from build123d import *

# Parameters (mm, degrees)
BOSS_EXTRUDE1_DEPTH         = 3.175
M3_CLEARANCE_HOLE1_D        = 3.6
F_1_4_CLEARANCE_HOLE1_D     = 7.14248
CUT_EXTRUDE1_DEPTH          = 640.11012417
F_8_CLEARANCE_HOLE1_D       = 4.9149
SKETCH15_R                  = 1.55
CUT_EXTRUDE2_DEPTH          = 640.11012417
SKETCH16_R                  = 3.3782
CUT_EXTRUDE3_DEPTH          = 640.11012417
FILLET1_R                   = 1
CUT_EXTRUDE4_DEPTH          = 640.088878697
FILLET2_R                   = 1.5
F_13_0_185_DIAMETER_HOLE1_D = 4.699
F_1_4_CLEARANCE_HOLE2_D     = 6.7564


with BuildPart() as part:
    # Sketch1 → Boss-Extrude1 (new, symmetric)
    with BuildSketch(Plane(origin=(0, 0, 0), x_dir=(1, 0, 0), z_dir=(0, 1, 0))):
        Polygon((0, -94.3735), (0, 94.3735), (-621.526239041, 148.75), (-621.526239041, -148.75), align=None)
    extrude(amount=BOSS_EXTRUDE1_DEPTH, both=True)

    # M3 Clearance Hole1 (through all)
    with Locations(Plane(origin=(0, 3.175, 0), x_dir=(1, 0, 0), z_dir=(0, 1, 0))):
        with Locations((-379.222, 34.29), (-384.81, 34.29), (-384.81, -34.29)):
            Hole(M3_CLEARANCE_HOLE1_D / 2)

    # 1/4 Clearance Hole1 (through all)
    with Locations(Plane(origin=(0, 3.175, 0), x_dir=(1, 0, 0), z_dir=(0, 1, 0))):
        with Locations((-29.147346667, 72.452653333), (-29.147346667, -72.452653333), (-148.652653333, -72.452653333), (-148.652653333, 72.452653333)):
            Hole(F_1_4_CLEARANCE_HOLE1_D / 2)

    # Sketch12 → Cut-Extrude1 (cut, through all)
    with BuildSketch(Plane(origin=(0, 3.175, 0), x_dir=(1, 0, 0), z_dir=(0, 1, 0))):
        with BuildLine():
            Line((-380.84125, -33.6169), (-380.84125, -34.0868))
            ThreePointArc((-380.84125, -34.0868), (-380.85395, -34.29), (-380.84125, -34.4932))
            Line((-380.84125, -34.4932), (-380.84125, -34.9631))
            ThreePointArc((-380.84125, -34.9631), (-379.222, -36.58235), (-377.60275, -34.9631))
            Line((-377.60275, -34.9631), (-377.60275, -34.4932))
            ThreePointArc((-377.60275, -34.4932), (-377.59005, -34.29), (-377.60275, -34.0868))
            Line((-377.60275, -34.0868), (-377.60275, -33.6169))
            ThreePointArc((-377.60275, -33.6169), (-379.222, -31.99765), (-380.84125, -33.6169))
        make_face()
    extrude(amount=-CUT_EXTRUDE1_DEPTH, mode=Mode.SUBTRACT)

    # #8 Clearance Hole1 (through all)
    with Locations(Plane(origin=(0, 3.175, 0), x_dir=(1, 0, 0), z_dir=(0, 1, 0))):
        with Locations((-508.833140591, -78.064272283), (-508.833140591, -103.464272283), (-543.213396712, -112.444528404), (-534.233140591, -78.064272283), (-481.407885674, -78.064272283), (-481.407885674, -103.464272283), (-456.007885674, -78.064272283), (-456.007885674, -103.464272283), (-456.007885674, 78.064272283), (-456.007885674, 103.464272283), (-481.407885674, 78.064272283), (-481.407885674, 103.464272283), (-543.213396712, 112.444528404), (-534.233140591, 78.064272283), (-508.833140591, 103.464272283), (-508.833140591, 78.064272283)):
            Hole(F_8_CLEARANCE_HOLE1_D / 2)

    # Sketch15 → Cut-Extrude2 (cut, through all)
    with BuildSketch(Plane(origin=(0, 3.175, 0), x_dir=(1, 0, 0), z_dir=(0, 1, 0))):
        with Locations(Location((-295.918163181, -81.916960017, 0), (0, 0, 270))):
            Circle(SKETCH15_R)
        with Locations(Location((-364.1575, -87.887128395, 0), (0, 0, 270))):
            Circle(SKETCH15_R)
    extrude(amount=-CUT_EXTRUDE2_DEPTH, mode=Mode.SUBTRACT)

    # Sketch16 → Cut-Extrude3 (cut, through all)
    with BuildSketch(Plane(origin=(0, 3.175, 0), x_dir=(1, 0, 0), z_dir=(0, 1, 0))):
        with Locations(Location((-609.6000104, -121.650317511, 0), (0, 0, 270))):
            Circle(SKETCH16_R)
        with Locations(Location((-609.6000104, -86.943080709, 0), (0, 0, 270))):
            Circle(SKETCH16_R)
        with Locations(Location((-609.6000104, 86.943080709, 0), (0, 0, 270))):
            Circle(SKETCH16_R)
        with Locations(Location((-609.6000104, 121.650317511, 0), (0, 0, 270))):
            Circle(SKETCH16_R)
    extrude(amount=-CUT_EXTRUDE3_DEPTH, mode=Mode.SUBTRACT)

    # Fillet1
    fillet1_edges = [part.edges().sort_by_distance(p)[0] for p in [
        (-621.526239041, 0, 148.75),
        (-621.526239041, 0, -148.75),
    ]]
    fillet(fillet1_edges, radius=FILLET1_R)

    # Sketch17 → Cut-Extrude4 (cut, through all)
    with BuildSketch(Plane(origin=(0, 3.175, 0), x_dir=(1, 0, 0), z_dir=(0, 1, 0))):
        Polygon((-3, 94.635965991), (-3, 59.635965991), (0, 59.635965991), (0, 94.3735), align=None)
    cut_extrude4 = extrude(amount=-CUT_EXTRUDE4_DEPTH, mode=Mode.SUBTRACT)

    # Mirror1: Cut-Extrude4 across plane
    add(cut_extrude4.mirror(Plane.XY), mode=Mode.SUBTRACT)

    # Fillet2
    fillet2_edges = [part.edges().sort_by_distance(p)[0] for p in [
        (0, 0, -59.635965991),
        (-3, 0, -59.635965991),
        (-3, 0, -94.635965991),
        (0, 0, 59.635965991),
        (-3, 0, 59.635965991),
        (-3, 0, 94.635965991),
    ]]
    fillet(fillet2_edges, radius=FILLET2_R - 0.0001)  # a hair under: the kernel refuses the full size

    # #13 (0.185) Diameter Hole1 (through all)
    with Locations(Plane(origin=(0, 3.175, 0), x_dir=(1, 0, 0), z_dir=(0, 1, 0))):
        with Locations((-354.44558465, 73.187743603), (-304.635849746, 68.829956465)):
            Hole(F_13_0_185_DIAMETER_HOLE1_D / 2)

    # 1/4 Clearance Hole2 (through all)
    with Locations(Plane(origin=(0, 3.175, 0), x_dir=(1, 0, 0), z_dir=(0, 1, 0))):
        with Locations((-14.732, 88.469940408), (-14.0462, -87.453940528), (-303.7332, 0)):
            Hole(F_1_4_CLEARANCE_HOLE2_D / 2)


solid = part.part
Build history of the part. All positions in model axes, mm. Round coordinates to 2 decimals unless told otherwise and drop trailing zeros. Loops run counter-clockwise (first coordinate to the right, second up) from the corner with the lowest first, then second, coordinate; pieces in that order, holes last. Notation, with made-up numbers: (31.25, 14.25) -> (63.25, 14.25) arc R23 cw to (63.25, 39.25) -> close; hole circle Ø3 at (-7, 26.5). An arc over 180 degrees is marked (long way). Use CSV: the item, a comma, the result in double quotes. Start each with the question number.
Q1. Saw through at A-A on y = -0.5. Count the separate pieces of the cut face and the enclosed holes in it, and give its area (3 significant figures).
Q2. Drill centre lines: L1, parallel to X at y = 0, z = 35.5; L2, parallel to Z at x = -131, y = 1; L3, parallel to Z at x = -286.5, y = 2.5. Where is each one in solid material? Low to high.
Q3. Flat gauge pins, fed straight in: pin 1 Ø2 at (x, y) = (-70.5, -2) entering from +Z; pin 2 Ø8 at (x, z) = (-481.41, 78.06) entering from -Y (3 decimals); pin 3 Ø3 at (x, y) = (-515.5, -0.5) entering from -Z; pin 4 Ø3 at (y, z) = (0, -81.5) entering from +X. Where does each tip first touch, or does it go through?
Q4. Mould opens along X. For faces 1 (the face through (-316.717, 0.044, 122.083)), 2 (the face through (-315, 3.175, -2)) say: +X half, -X half, draft (parallel to the pull), parting line (faces both ways), or undercut.
Q5. Saw through at B-B on x = -243. Give the cut face in (y, z) (3 decimals), and give its area (3 significant figures).
Solutions:
1,separate pieces,"1"
1,enclosed holes,"35"
1,area,"150,000 mm^2"
2,L1,"x = -621.53 to -386.14, -383.48 to -380.75, -377.69 to 0"
2,L2,"z = -105.83 to 105.83"
2,L3,"z = -119.44 to 119.44"
3,pin 1,"stops at z = 100.63"
3,pin 2,"stops at y = -3.175"
3,pin 3,"stops at z = -139.61"
3,pin 4,"stops at x = -3"
4,face 1,"+X half"
4,face 2,"draft"
5,outline,"(-3.175, -115.633) -> (3.175, -115.633) -> (3.175, 115.633) -> (-3.175, 115.633) -> close"
5,area,"1,470 mm^2"
